```python
from build123d import *

# Parameters (mm, degrees)
SKETCH1_R           = 2
SKETCH1_R_2         = 15
BOSS_EXTRUDE1_DEPTH = 5


with BuildPart() as part:
    # Sketch1 → Boss-Extrude1 (new body)
    with BuildSketch(Plane(origin=(0, 0, 0), x_dir=(1, 0, 0), z_dir=(0, 1, 0))):
        Polygon((-63.5, 9), (-53.5, 19), (21, 19), (31, 9), (31, -9), (21, -19), (-53.5, -19), (-63.5, -9), align=None)
        with Locations(Location((-25, 0, 0), (0, 0, 270))):
            Circle(SKETCH1_R, mode=Mode.SUBTRACT)
        with Locations(Location((25, 0, 0), (0, 0, 270))):
            Circle(SKETCH1_R, mode=Mode.SUBTRACT)
        with Locations(Location((0, 0, 0), (0, 0, 270))):
            Circle(SKETCH1_R_2, mode=Mode.SUBTRACT)
        with BuildLine():
            Line((-57.5, 2), (-42.5, 2))
            ThreePointArc((-42.5, 2), (-40.5, 0), (-42.5, -2))
            Line((-42.5, -2), (-57.5, -2))
            ThreePointArc((-57.5, -2), (-59.5, 0), (-57.5, 2))
        make_face(mode=Mode.SUBTRACT)
    extrude(amount=-BOSS_EXTRUDE1_DEPTH)


solid = part.part
```
Check sheet for the modelled part. Datum: model origin and axes. Units: mm. A direction names the side the tool comes from. Round coordinates to 2 decimals unless told otherwise and drop trailing zeros. Write each loop counter-clockwise with the first axis right and the second up, starting at its lowest first coordinate (ties: lowest second). Pieces come first, ordered by that corner, then holes. Notation, with made-up numbers: (-33, 49) -> (21, 49) arc R23 cw to (21, 85) -> close; hole circle Ø5 at (82, 33). An arc over 180 degrees is marked (long way). One line per question, with ' | ' between items. Start each with the question number.
1. Sectioned sample at C-C, the plane y = -1.3. Record the cut outline in (x, z), then the cut area to 3 significant figures.
2. Depth check by flat-ended pin: pin 1 (2.5 mm diameter, centred on x = -25, z = 0, fed in from +Y). Enter the tip coordinate at first touch or a pass-through.
3. Sectioned sample at A-A, the plane z = 0. Record the cut outline in (x, y), then the cut area to 4 significant figures.
4. Set-up check for faces 1 (the face through (31, -2, 0)), 2 (the face through (-59.5, -2.5, 0)): record each of +Z, -Z, +X, -X, +Y, -Y from which the full face is reachable in a straight line by a thin tool's end or side.
5. Scan lines: line 1 along X through (y, z) = (-2.2, 0); line 2 along Z through (x, y) = (-0.5, -3.85); line 3 along Z through (x, y) = (-7, -2.5). Record each from-to range of solid material in increasing order. Write a range as from..to.
6. Release check for a two-part mould opening along Z. For faces 3 (the face through (-16, -2, 19)), 4 (the face through (-58.6, -2.5, -13.9)), 5 (the face through (-26.2, -2.5, -1.6)) record: +Z half, -Z half, draft (parallel to the pull), parting line (faces both ways), or undercut.
7. Sectioned sample at D-D, the plane z = -7.5. Record the cut outline in (x, y).
8. Sectioned sample at B-B, the plane x = 0. Record the cut outline in (y, z).
Taken from the geometry:
1) outline: (-63.5, -9) -> (-53.5, -19) -> (21, -19) -> (31, -9) -> (31, 9) -> (21, 19) -> (-53.5, 19) -> (-63.5, 9) -> close; hole (-57.5, -2) -> (-42.5, -2) arc R2 ccw to (-42.5, 2) -> (-57.5, 2) arc R2 ccw to start; hole circle Ø4 at (-25, 0); hole circle Ø30 at (0, 0); hole circle Ø4 at (25, 0) | area: 2,590 mm^2
2) pin 1: passes through
3) outline: (-63.5, -5) -> (-59.5, -5) -> (-59.5, 0) -> (-63.5, 0) -> close; (-40.5, -5) -> (-27, -5) -> (-27, 0) -> (-40.5, 0) -> close; (-23, -5) -> (-15, -5) -> (-15, 0) -> (-23, 0) -> close; (15, -5) -> (23, -5) -> (23, 0) -> (15, 0) -> close; (27, -5) -> (31, -5) -> (31, 0) -> (27, 0) -> close | area: 187.5 mm^2
4) face 1: +Z, -Z, +X, +Y, -Y | face 2: +Y, -Y
5) line 1: x = -63.5..-59.5, -40.5..-27, -23..-15, 15..23, 27..31 | line 2: z = -19..-14.99, 14.99..19 | line 3: z = -19..-13.27, 13.27..19
6) face 3: +Z half | face 4: -Z half | face 5: undercut
7) outline: (-63.5, -5) -> (-12.99, -5) -> (-12.99, 0) -> (-63.5, 0) -> close; (12.99, -5) -> (31, -5) -> (31, 0) -> (12.99, 0) -> close
8) outline: (-5, -19) -> (0, -19) -> (0, -15) -> (-5, -15) -> close; (-5, 15) -> (0, 15) -> (0, 19) -> (-5, 19) -> close
